from build123d import *

# Parameters (mm, degrees)
F0_R     = 2
F1_DEPTH = 4


with BuildPart() as f1:
    # F0 (on Front) → F1 (new body)
    with BuildSketch(Plane.XZ):
        Polygon((32, -32), (32, 32), (17.497475, 17.497475), (3.355339, 31.63961), (-32, -3.715729), (-17.857864, -17.857864), (-32, -32), (-26, -32), (-26, -42), (-6, -42), (-6, -32), (6, -32), (6, -42), (26, -42), (26, -32), align=None)
        with Locations((-6.859445, 9.531957)):
            Circle(F0_R, mode=Mode.SUBTRACT)
        with Locations((10.066459, -3.652432)):
            Circle(F0_R, mode=Mode.SUBTRACT)
    extrude(amount=F1_DEPTH)


solid = f1.part
The listing builds one solid part. Answer for the finished solid, in the listing's coordinates (mm). A direction names the side the tool comes from. Round coordinates to 2 decimals unless told otherwise and drop trailing zeros. Write each loop counter-clockwise with the first axis right and the second up, starting at its lowest first coordinate (ties: lowest second). Pieces come first, ordered by that corner, then holes. Notation, with made-up numbers: (6, 60) - (57, 60) arc R20 ccw to (57, 93) - close; hole circle Ø8 at (-26, 5.5). An arc over 180 degrees is marked (long way). Use one line per item in the form item = value. Start each with the question number.
Item 1: A cutting plane is placed at D-D (z = -22.5). Write down the section's boundary in (x, y), plus the area to 3 significant figures.
Item 2: A tool of negligible diameter and unlimited length cuts with its end or side. For faces 1 (the flat face through (10.525, -1.972, 24.47)), 2 (the flat face through (29, -2, -32)), 3 (the flat face through (6, -2, -37)), 4 (the flat face through (-25, -2, -25)), 5 (the flat face through (-26, -2, -37)), from which of +Z, -Z, +X, -X, +Y, -Y can it reach the whole face along a straight path? Write none if from no direction.
Item 3: Flat-ended cylindrical pins translate along their axes: pin 1 Ø2 at (y, z) = (-2.5, -39.5) entering from -X; pin 2 Ø2 at (y, z) = (-1, -37.5) entering from +X; pin 3 Ø1.2 at (x, y) = (0, -3) entering from -Z; pin 4 Ø2.5 at (x, z) = (10.07, -3.65) entering from +Y. Find the tip coordinate at first contact, or state that the pin passes through.
Item 4: Find the intervals of material crossed by line 1 (X direction, y = -1.35, z = -34.5); line 2 (X direction, y = -1.5, z = 26); line 3 (Z direction, x = -8, y = -1.75), in increasing order. Write a range as [from, to].
Item 5: Determine the mould class of faces 6 (the flat face through (-25.028, -1.972, -10.688)), 7 (the flat face through (-29, -2, -32)), 8 (the flat face through (26, -2, -37)), 9 (the flat face through (25, -2, 25)) for opening direction X: +X half, -X half, draft (parallel to the pull), parting line (faces both ways), or undercut.
Item 6: A cutting plane is placed at B-B (z = -33.5). Write down the section's boundary in (x, y).
Item 7: A cutting plane is placed at A-A (x = -28). Write down the section's boundary in (y, z), plus the area to 3 significant figures.
Item 8: A cutting plane is placed at C-C (y = -2). Write down the section's boundary in (x, z).
The answers:
q1.outline = (-22.5, -4) - (32, -4) - (32, 0) - (-22.5, 0) - close
q1.area = 218 mm^2
q2.face_1 = +Z, +Y, -Y
q2.face_2 = -Z, +X, +Y, -Y
q2.face_3 = -Z, +Y, -Y
q2.face_4 = -X, +Y, -Y
q2.face_5 = -Z, -X, +Y, -Y
q3.pin_1 = -26
q3.pin_2 = 26
q3.pin_3 = -32
q3.pin_4 = through
q4.line_1 = [-26, -6], [6, 26]
q4.line_2 = [-2.28, 8.99], [26, 32]
q4.line_3 = [-42, 7.89], [11.17, 20.28]
q5.face_6 = -X half
q5.face_7 = draft
q5.face_8 = +X half
q5.face_9 = undercut
q6.outline = (-26, -4) - (-6, -4) - (-6, 0) - (-26, 0) - close; (6, -4) - (26, -4) - (26, 0) - (6, 0) - close
q7.outline = (-4, -32) - (0, -32) - (0, -28) - (-4, -28) - close; (-4, -7.72) - (0, -7.72) - (0, 0.28) - (-4, 0.28) - close
q7.area = 48.0 mm^2
q8.outline = (-32, -32) - (-26, -32) - (-26, -42) - (-6, -42) - (-6, -32) - (6, -32) - (6, -42) - (26, -42) - (26, -32) - (32, -32) - (32, 32) - (17.5, 17.5) - (3.36, 31.64) - (-32, -3.72) - (-17.86, -17.86) - close; hole circle Ø4 at (-6.86, 9.53); hole circle Ø4 at (10.07, -3.65)
